Source: CAD feature listing. Evaluate the final solid. Frame: model axes, mm. Face numbers are marked on the shaded views. A direction names the side the tool comes from. Give positions to 0.01 mm unless a question says otherwise; leave off trailing zeros. Write each loop counter-clockwise with the first axis right and the second up, starting at its lowest first coordinate (ties: lowest second). Pieces come first, ordered by that corner, then holes. Notation, with made-up numbers: M -24.75,16 L 32.25,16 A25 cw 32.25,35 Z; hole C -11.5,31 d8. An arc over 180 degrees is marked long. Answer as a JSON object with one key per item and string values. Group by question number.
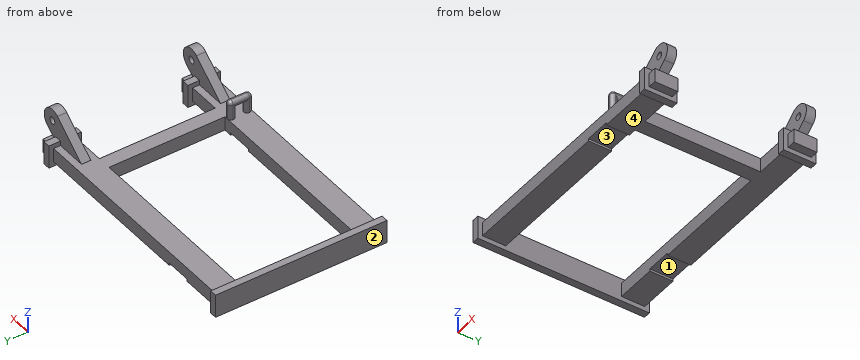
```python
from build123d import *

# Parameters (mm, degrees)
F0_W          = 1.524
F0_H          = 12.7
F1_DEPTH      = 1.524
F2_W          = 0.762
F2_H          = 18.796
F2_H_2        = 3.556
F3_DEPTH      = 0.508
F3_DEPTH_BACK = 2.032
F4_R          = 0.381
F5_DEPTH      = 1.778
F7_DEPTH      = 0.762
F9_W          = 2.794
F9_H          = 2.54
F10_DEPTH     = 0.254
F11_W         = 2.54
F11_H         = 1.524
F12_DEPTH     = 0.889
F13_W         = 2.54
F13_H         = 1.524
F14_DEPTH     = 0.889
F15_W         = 0.762
F15_H         = 0.762
F16_DEPTH     = 2.032
F17_W         = 0.762
F17_H         = 0.762
F18_DEPTH     = 1.016
F19_R         = 0.38099


# Not quite as in the source:
# - a fillet or chamfer is up to 0.001 mm smaller than in the source, because OpenCascade refuses the exact size
# - a pattern or mirror of a feature is missing from the dataset's text; its kind, count and spacing are read off the source's solid


with BuildPart() as f1:
    # F0 (on Top) → F1 (new body)
    with BuildSketch(Plane.XY):
        Polygon((-12.7, 17.78), (-12.7, 15.24), (7.62, 15.24), (9.144, 15.24), (12.7, 15.24), (12.7, 17.78), align=None)
        Polygon((-12.7, 0), (-12.7, 2.54), (-12.7, 15.24), (-12.7, 17.78), (-12.7, 18.288), (-13.462, 18.288), (-13.462, -0.508), (-12.7, -0.508), align=None)
        Polygon((7.62, 2.54), (-12.7, 2.54), (-12.7, 0), (12.7, 0), (12.7, 2.54), (9.144, 2.54), align=None)
        with Locations((8.382, 8.89)):
            Rectangle(F0_W, F0_H)
        Polygon((12.7, 2.54), (12.7, 0), (12.7, -0.508), (13.462, -0.508), (13.462, 3.048), (12.7, 3.048), align=None)
        Polygon((12.7, 18.288), (12.7, 17.78), (12.7, 15.24), (12.7, 14.732), (13.462, 14.732), (13.462, 18.288), align=None)
    extrude(amount=F1_DEPTH)

    # F2 (on face) → F3 (join, two sides)
    with BuildSketch(Plane.XY.offset(1.524)) as f3_sk:
        with Locations((-13.081, 8.89)):
            Rectangle(F2_W, F2_H)
        with Locations((13.081, 16.51)):
            Rectangle(F2_W, F2_H_2)
        with Locations((13.081, 1.27)):
            Rectangle(F2_W, F2_H_2)
    extrude(amount=F3_DEPTH)
    extrude(f3_sk.sketch, amount=-F3_DEPTH_BACK)

    # F4 (on face) → F5 (join)
    with BuildSketch(Plane.XZ):
        with BuildLine():
            Line((13.462, 1.524), (14.762993756, 2.564001561))
            ThreePointArc((14.762993756, 2.564001561), (14.961998439, 4.348993756), (13.177006244, 4.547998439))
            Line((13.177006244, 4.547998439), (9.3941243381, 1.524))
            Line((9.3941243381, 1.524), (13.462, 1.524))
        make_face()
        with Locations((13.97, 3.556)):
            Circle(F4_R, mode=Mode.SUBTRACT)
    f5 = extrude(amount=-F5_DEPTH)

    # F5_copies: F5 across plane
    add(f5.mirror(Plane.ZX.offset(8.89)))

    # F6 (on face) → F7 (cut)
    with BuildSketch(Plane.XZ):
        with BuildLine():
            Line((13.177006244, 4.547998439), (9.3941243381, 1.524))
            Line((9.3941243381, 1.524), (12.7, 1.524))
            Line((12.7, 1.524), (12.7, 2.032))
            Line((12.7, 2.032), (13.462, 2.032))
            Line((13.462, 2.032), (13.462, 1.524))
            Line((13.462, 1.524), (14.762993756, 2.564001561))
            ThreePointArc((14.762993756, 2.564001561), (14.961998439, 4.348993756), (13.177006244, 4.547998439))
        make_face()
    f7 = extrude(amount=-F7_DEPTH, mode=Mode.SUBTRACT)

    # F7_copies: F7 across plane
    add(f7.mirror(Plane.ZX.offset(8.89)), mode=Mode.SUBTRACT)

    # F9 (on face) → F10 (cut)
    with BuildSketch(Plane(origin=(0, 0, 0), x_dir=(1, 0, 0), z_dir=(0, 0, -1))):
        with Locations((5.334, -1.27)):
            Rectangle(F9_W, F9_H)
        with Locations((-6.858, -16.51)):
            Rectangle(F9_W, F9_H)
    extrude(amount=-F10_DEPTH, mode=Mode.SUBTRACT)

    # F11 (on face) → F12 (join)
    with BuildSketch(Plane.YZ.offset(13.462)):
        with Locations((1.27, 0.762)):
            Rectangle(F11_W, F11_H)
    extrude(amount=F12_DEPTH)

    # F13 (on face) → F14 (join)
    with BuildSketch(Plane.YZ.offset(13.462)):
        with Locations((16.51, 0.762)):
            Rectangle(F13_W, F13_H)
    extrude(amount=F14_DEPTH)

    # F15 (on face) → F16 (join)
    with BuildSketch(Plane.XY.offset(1.524)):
        with Locations((7.239, 2.159)):
            Rectangle(F15_W, F15_H)
        with Locations((7.239, 0.381)):
            Rectangle(F15_W, F15_H)
    extrude(amount=F16_DEPTH)

    # F17 (on face) → F18 (join, through all)
    with BuildSketch(Plane.XZ.offset(-1.778)):
        with Locations((7.239, 3.175)):
            Rectangle(F17_W, F17_H)
    extrude(amount=F18_DEPTH)

    # F19 (radius 0.381 in the source; OpenCascade refuses exactly that, so slightly less here)
    f19_edges = [f1.edges().sort_by_distance(p)[0] for p in [
        (6.858, 2.54, 2.54),
        (7.62, 2.54, 2.54),
        (7.239, 2.54, 3.556),
        (7.62, 1.27, 3.556),
        (6.858, 1.27, 3.556),
        (6.858, 1.27, 2.794),
        (6.858, 1.778, 2.159),
        (6.858, 0.762, 2.159),
        (7.62, 0.762, 2.159),
        (6.858, 0, 2.54),
        (7.239, 0, 3.556),
        (7.62, 1.27, 2.794),
        (7.62, 0, 2.54),
        (7.62, 1.778, 2.159),
    ]]
    fillet(f19_edges, radius=F19_R)


solid = f1.part
```
(1) Access query for the marked faces 1, 2, 3 and 4. Directions: +Z, -Z, +X, -X, +Y, -Y. A direction counts if a zero-diameter tool reaches every point of the face in a straight line with its end or side. Return the directions, or none.
(2) Section B-B, the plane y = 9. Return loops of the section in (x, z), plus the area to 3 significant figures.
(3) Contact query for flat-ended pins moving along their axis: pin 1 Ø1 at (x, z) = (9, 0) entering from -Y; pin 2 Ø3 at (x, y) = (5, 5.5) entering from -Z; pin 3 Ø1.8 at (y, z) = (1, 2.5) entering from +X; pin 4 Ø3 at (y, z) = (12.5, 2) entering from +X. Output: stop coordinate, or through.
(4) Ray query, L1, parallel to X at y = 6, z = 1.15; L2, parallel to X at y = 17, z = -0.3; L3, parallel to Y at x = -3.75, z = 1. Return the intervals inside material, ascending. Write a range as [from, to].
(5) Section A-A, the plane x = -0.5. Return loops of the section in (y, z).
(6) Section D-D, the plane x = 13.97. Return loops of the section in (y, z) (3 decimals), plus the area to 3 significant figures.
Reported:
{
 "1": {"face 1": "-Z, +Y", "face 2": "+Z, -Z, -X, +Y, -Y", "face 3": "-Z, -Y", "face 4": "-Z, +Y, -Y"},
 "2": {"outline": "M -13.46,-0.51 L -12.7,-0.51 L -12.7,2.03 L -13.46,2.03 Z; M 7.62,0 L 9.14,0 L 9.14,1.52 L 7.62,1.52 Z", "area": "4.26 mm2"},
 "3": {"pin 1": "stops at y = 0", "pin 2": "passes through", "pin 3": "stops at x = 15.23", "pin 4": "stops at x = 9.14"},
 "4": {"L1": "x = [-13.46, -12.7], [7.62, 9.14]", "L2": "x = [-13.46, -12.7], [12.7, 13.46]", "L3": "y = [0, 2.54], [15.24, 17.78]"},
 "5": {"outline": "M 0,0 L 2.54,0 L 2.54,1.52 L 0,1.52 Z; M 15.24,0 L 17.78,0 L 17.78,1.52 L 15.24,1.52 Z"},
 "6": {"outline": "M 0,0 L 2.54,0 L 2.54,1.524 L 0,1.524 Z; M 0.762,1.93 L 1.778,1.93 L 1.778,3.175 L 0.762,3.175 Z; M 0.762,3.937 L 1.778,3.937 L 1.778,4.826 L 0.762,4.826 Z; M 15.24,0 L 17.78,0 L 17.78,1.524 L 15.24,1.524 Z; M 16.002,1.93 L 17.018,1.93 L 17.018,3.175 L 16.002,3.175 Z; M 16.002,3.937 L 17.018,3.937 L 17.018,4.826 L 16.002,4.826 Z", "area": "12.1 mm2"}
}
